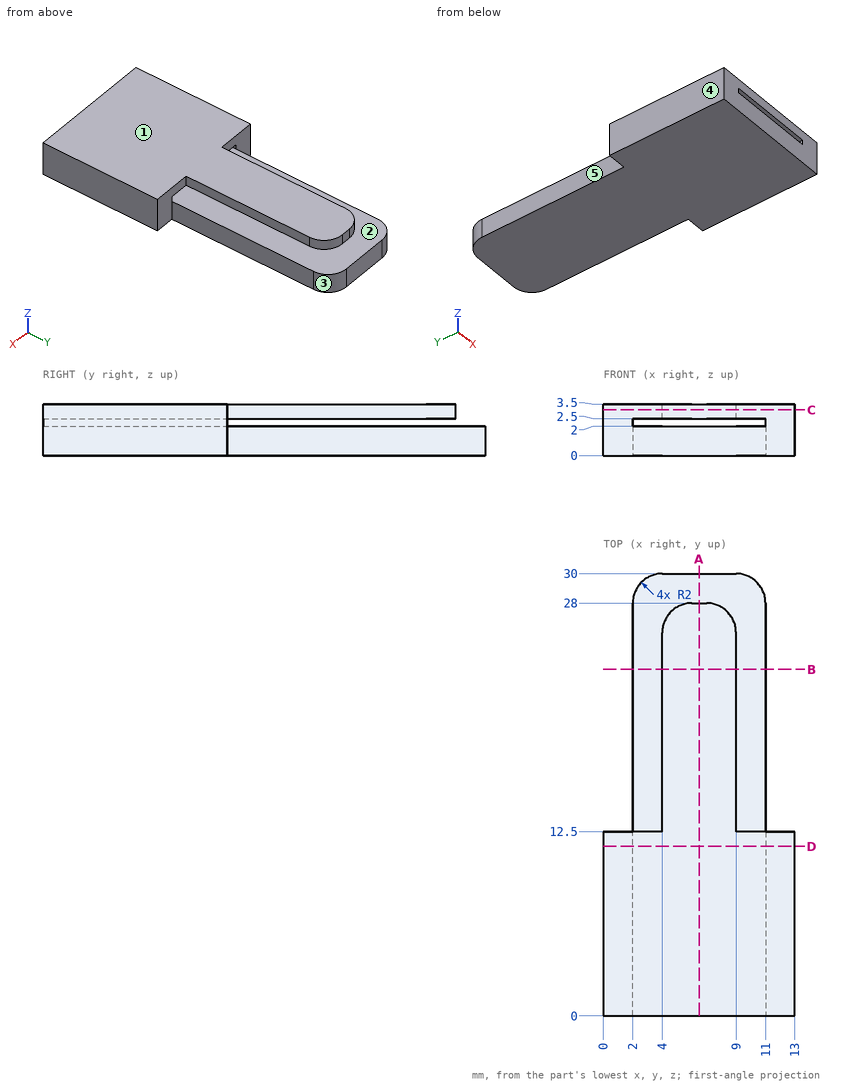
Input: dimensioned drawing with shaded views. Units: mm. Origin: part minimum x, y, z. A direction names the side the tool comes from. Coordinates: 2 decimals unless noted, no trailing zeros. Order: outer loops, then holes, each group sorted by start corner. A loop starts at its lowest first (then second) coordinate and runs counter-clockwise, first axis right, second up. Notation, with made-up numbers: (31, 15.25) -> (61, 15.25) arc R27 ccw to (61, 45.25) -> close; hole circle Ø7 at (-31, -9.5). An arc over 180 degrees is marked (long way). Use CSV: the item, a comma, the result in double quotes.
1) Pin query (flat end, axial travel): pin 1 Ø1.5 at (x, z) = (10.5, 1.5) entering from +Y; pin 2 Ø1.1 at (y, z) = (20.5, 3) entering from -X; pin 3 Ø1 at (y, z) = (19.5, 2) entering from +X. Return the tip coordinate at first contact, or that it passes through.
Findings:
pin 1,"stops at y = 29.85"
pin 2,"stops at x = 4"
pin 3,"stops at x = 11"
2) Mould query, pull axis X, two halves, no side actions, for the marked faces 1, 2 and 3. Classes: +X half, -X half, draft (parallel to the pull), parting line (faces both ways), or undercut.
Findings:
face 1,"draft"
face 2,"undercut"
face 3,"+X half"
3) Section A-A on x = 6.5. Output: boundary loops of the cut face in (y, z), then the cut area to 3 significant figures.
Findings:
outline,"(0, 0) -> (30, 0) -> (30, 2) -> (0, 2) -> close; (0, 2.5) -> (28, 2.5) -> (28, 3.5) -> (0, 3.5) -> close"
area,"88.0 mm^2"
4) Access query for the marked faces 4 and 5. Directions: +Z, -Z, +X, -X, +Y, -Y. A direction counts if a zero-diameter tool reaches every point of the face in a straight line with its end or side. Return the directions, or none.
Findings:
face 4,"+Z, -Z, -X, +Y, -Y"
face 5,"+Z, -Z, -X, +Y"
5) Section D-D on y = 11.5. Output: boundary loops of the cut face in (x, z).
Findings:
outline,"(0, 0) -> (13, 0) -> (13, 3.5) -> (0, 3.5) -> close; hole (2, 2) -> (11, 2) -> (11, 2.5) -> (2, 2.5) -> close"
6) Section C-C on z = 3.1. Output: boundary loops of the cut face in (x, y), then the cut area to 3 significant figures.
Findings:
outline,"(0, 0) -> (13, 0) -> (13, 12.5) -> (9, 12.5) -> (9, 26) arc R2 ccw to (7, 28) -> (6, 28) arc R2 ccw to (4, 26) -> (4, 12.5) -> (0, 12.5) -> close"
area,"238 mm^2"
7) Section B-B on y = 23.5. Output: boundary loops of the cut face in (x, z).
Findings:
outline,"(2, 0) -> (11, 0) -> (11, 2) -> (2, 2) -> close; (4, 2.5) -> (9, 2.5) -> (9, 3.5) -> (4, 3.5) -> close"
8) Line query: line 1 (Z direction, x = 8.5, y = 16.5); line 2 (X direction, y = 20.25, z = 2.9); line 3 (Y direction, x = 9.25, z = 2.65). Output: solid intervals per line, ascending.
Findings:
line 1,"z = 0 to 2, 2.5 to 3.5"
line 2,"x = 4 to 9"
line 3,"y = 0 to 12.5"
